from build123d import *

# Parameters (mm, degrees)
BOSS_EXTRUDE2_DEPTH = 25.4
SKETCH6_W           = 29.894889523
SKETCH6_H           = 12.7
CUT_EXTRUDE2_DEPTH  = 25.4
SKETCH7_W           = 29.894889523
SKETCH7_H           = 12.7
CUT_EXTRUDE3_DEPTH  = 25.4
SKETCH8_W           = 29.894889523
SKETCH8_H           = 12.7
CUT_EXTRUDE4_DEPTH  = 25.4
SKETCH9_R           = 2.625984609
CUT_EXTRUDE5_DEPTH  = 25.4


with BuildPart() as part:
    # Sketch5 → Boss-Extrude2 (new body)
    with BuildSketch(Plane(origin=(0, 0, 0), x_dir=(1, 0, 0), z_dir=(0, 1, 0))):
        with BuildLine():
            Line((0.906871592, 19.028402033), (7.829859105, 17.366513939))
            ThreePointArc((7.829859105, 17.366513939), (29.524645576, 0.411973336), (42.722311342, -23.75291494))
            ThreePointArc((42.722311342, -23.75291494), (30.571840916, -14.649217341), (16.025643758, -10.299574853))
            Line((16.025643758, -10.299574853), (11.124912694, -15.464113863))
            ThreePointArc((11.124912694, -15.464113863), (-14.405543413, -25.775079775), (-41.931783423, -25.12214946))
            ThreePointArc((-41.931783423, -25.12214946), (-27.972514821, -19.151382203), (-16.93251535, -8.72882718))
            Line((-16.93251535, -8.72882718), (-18.954771799, -1.902400076))
            ThreePointArc((-18.954771799, -1.902400076), (-15.119102163, 25.363106438), (-0.790527919, 48.8750644))
            ThreePointArc((-0.790527919, 48.8750644), (-2.599326095, 33.800599544), (0.906871592, 19.028402033))
        make_face()
    extrude(amount=BOSS_EXTRUDE2_DEPTH)

    # Sketch6 → Cut-Extrude2 (cut)
    with BuildSketch(Plane(origin=(1.982617129, 0, -0.112752753), x_dir=(-0.05677891901057157, 0, -0.9983867759320488), z_dir=(0.9983867759320488, 0, -0.05677891901057157))):
        with Locations((33.89365853, 12.7)):
            Rectangle(SKETCH6_W, SKETCH6_H)
    extrude(amount=-CUT_EXTRUDE2_DEPTH, mode=Mode.SUBTRACT)

    # Sketch7 → Cut-Extrude3 (cut)
    with BuildSketch(Plane(origin=(-0.893661816, 0, 1.773373176), x_dir=(0.8930177702648826, 0, 0.45002140170344945), z_dir=(-0.4500214017034494, 0, 0.8930177702648825))):
        with Locations((33.89365853, 12.7)):
            Rectangle(SKETCH7_W, SKETCH7_H)
    extrude(amount=-CUT_EXTRUDE3_DEPTH, mode=Mode.SUBTRACT)

    # Sketch8 → Cut-Extrude4 (cut)
    with BuildSketch(Plane(origin=(-1.088955313, 0, -1.660620423), x_dir=(-0.8362388512543109, 0, 0.5483653742285982), z_dir=(-0.5483653742285982, 0, -0.8362388512543109))):
        with Locations((33.89365853, 12.7)):
            Rectangle(SKETCH8_W, SKETCH8_H)
    extrude(amount=-CUT_EXTRUDE4_DEPTH, mode=Mode.SUBTRACT)

    # Sketch9 → Cut-Extrude5 (cut)
    with BuildSketch(Plane(origin=(0, 0, 0), x_dir=(1, 0, 0), z_dir=(0, 1, 0))):
        with Locations(Location((0, 0, 0), (0, 0, 270))):
            Circle(SKETCH9_R)
    extrude(amount=CUT_EXTRUDE5_DEPTH, mode=Mode.SUBTRACT)


solid = part.part
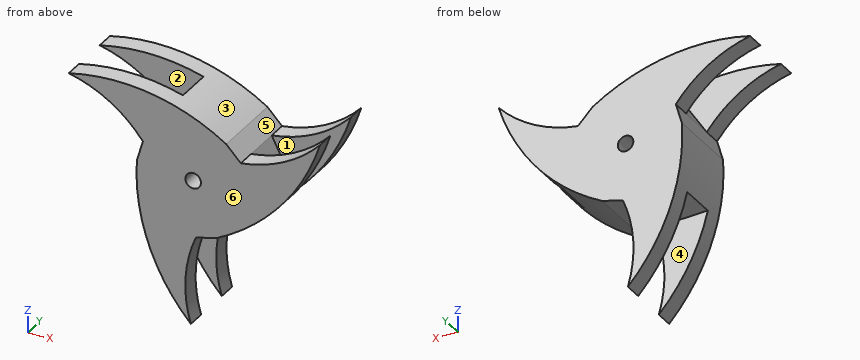
Geometry check sheet. Reference: the model listing, model coordinates, mm. Face numbers are marked on the shaded views. A direction names the side the tool comes from. Round coordinates to 2 decimals unless told otherwise and drop trailing zeros. Loops run counter-clockwise (first coordinate to the right, second up) from the corner with the lowest first, then second, coordinate; pieces in that order, holes last. Notation, with made-up numbers: (54.25, 22) - (81.25, 22) arc R28 ccw to (81.25, 54) - close; hole circle Ø8 at (78, 9). An arc over 180 degrees is marked (long way). One line per question, with ' | ' between items. Start each with the question number.
1. Cross-section at D-D on z = 0. Record the cut outline in (x, y), then the cut area to 3 significant figures.
2. Scan lines: line 1 (Y direction, x = -22, z = 23); line 2 (X direction, y = 12.25, z = 0); line 3 (X direction, y = 8.5, z = 1). Record each from-to range of solid material in increasing order. Write a range as [from, to].
3. Tool access check on the marked faces 1, 2 and 3. Record the directions out of +Z, -Z, +X, -X, +Y, -Y that give a thin tool (end or side, any length) a straight path to the whole face; none if there is none.
4. Cross-section at A-A on y = 23. Record the cut outline in (x, z), then the cut area to 3 significant figures.
5. Cross-section at C-C on x = 25.5. Record the cut outline in (y, z), then the cut area to 3 significant figures.
6. Cross-section at B-B on z = 22.5. Record the cut outline in (x, y).
7. Depth check by flat-ended pin: pin 1 (10 mm diameter, centred on y = 3.5, z = -11.5, fed in from +X); pin 2 (8 mm diameter, centred on y = 7, z = 0, fed in from -X); pin 3 (3 mm diameter, centred on x = 6.5, y = 5.5, fed in from +Z). Enter the tip coordinate at first touch or a pass-through.
8. Draft check along Y on the marked faces 4, 5 and 6. Enter one of: released by +Y, released by -Y, zero draft, split by the parting line, or undercut.
Taken from the geometry:
1) outline: (-19.05, 0) - (-2.63, 0) - (-2.63, 25.4) - (-19.05, 25.4) - close; (2.63, 0) - (29.87, 0) - (29.87, 6.35) - (21.22, 6.35) - (21.22, 19.05) - (29.87, 19.05) - (29.87, 25.4) - (2.63, 25.4) - close | area: 999 mm²
2) line 1: [0, 6.35], [19.05, 25.4] | line 2: [-19.05, -2.63], [2.63, 21.22] | line 3: [-19.01, -2.43], [2.43, 20.71]
3) face 1: +Z, +X | face 2: +Z, -X | face 3: +Z, +Y, -Y
4) outline: (-41.93, 25.12) arc R43.3 cw to (-16.93, 8.73) - (-18.95, 1.9) arc R68.03 ccw to (-0.79, -48.88) arc R43.3 cw to (0.91, -19.03) - (7.83, -17.37) arc R68.03 ccw to (42.72, 23.75) arc R43.3 cw to (16.03, 10.3) - (11.12, 15.46) arc R68.03 ccw to start; hole circle Ø5.25 at (0, 0) | area: 2,110 mm²
5) outline: (0, -4.76) - (6.35, -4.76) - (6.35, 12.49) - (0, 12.49) - close; (19.05, -4.76) - (25.4, -4.76) - (25.4, 12.49) - (19.05, 12.49) - close | area: 219 mm²
6) outline: (-34.11, 0) - (-2.59, 0) - (-2.59, 25.4) - (-34.11, 25.4) - (-34.11, 19.05) - (-7.9, 19.05) - (-7.9, 6.35) - (-34.11, 6.35) - close; (41.5, 0) - (42.33, 0) - (42.33, 6.35) - (41.5, 6.35) - close; (41.5, 19.05) - (42.33, 19.05) - (42.33, 25.4) - (41.5, 25.4) - close
7) pin 1: x = 23.67 | pin 2: x = -19.09 | pin 3: z = 19.1
8) face 4: undercut | face 5: zero draft | face 6: released by -Y
